The listing builds one solid part. Answer for the finished solid, in the listing's coordinates (mm). A direction names the side the tool comes from. Give positions to 0.01 mm unless a question says otherwise; leave off trailing zeros. Loops run counter-clockwise (first coordinate to the right, second up) from the corner with the lowest first, then second, coordinate; pieces in that order, holes last. Notation, with made-up numbers: (-15.5, -39) -> (43.5, -39) arc R20 cw to (43.5, -23) -> close; hole circle Ø11 at (-30, -15.5). An arc over 180 degrees is marked (long way). One line per question, with ' | ' between items. Start each with the question number.
from build123d import *

# Parameters (mm, degrees)
F1_DEPTH = 10
F2_R     = 10
F3_DEPTH = 10


with BuildPart() as f1:
    # F0 (on Front) → F1 (new body)
    with BuildSketch(Plane.XZ):
        Polygon((0, 10), (0, 0), (60, 0), (60, 10), (26.784621, 10), align=None)
        with BuildLine():
            ThreePointArc((23.443592, 24.368972), (23.75282, 16.867964), (26.784621, 10))
            Line((26.784621, 10), (60, 10))
            ThreePointArc((60, 10), (50.768452, 40.200275), (23.443592, 24.368972))
        make_face()
        with BuildLine():
            Line((0, 30), (0, 10))
            Line((0, 10), (26.784621, 10))
            ThreePointArc((26.784621, 10), (23.75282, 16.867964), (23.443592, 24.368972))
            ThreePointArc((23.443592, 24.368972), (15.503914, 24.276899), (10, 30))
            Line((10, 30), (0, 30))
        make_face()
    extrude(amount=F1_DEPTH)

    # F2 (on face) → F3 (cut)
    with BuildSketch(Plane.XZ.offset(10)):
        with Locations((43.884981, 25.819998)):
            Circle(F2_R)
    extrude(amount=-F3_DEPTH, mode=Mode.SUBTRACT)


solid = f1.part
1. Straight lines are drawn through the part: L1, parallel to X at y = -7.25, z = 27.5; L2, parallel to X at y = -1, z = 21; L3, parallel to X at y = -2.75, z = 31.5. For each, find the intervals that lie inside material, in ascending order.
2. The part is cut by section C-C (z = 6). Write down the section's boundary in (x, y).
3. The part is cut by section B-B (y = -8). Write down the section's boundary in (x, z), plus the area to 3 significant figures.
4. Determine the mould class of faces 1 (the cylindrical face through (15.61, -4.93, 24.233)), 2 (the cylindrical face through (51.24, -4.93, 40.01)), 3 (the flat face through (31, 0, 16)), 4 (the cylindrical face through (48.5, -5.07, 16.95)) for opening direction Z: released by +Z, released by -Z, zero draft, split by the parting line, or undercut.
5. Each of these flat-tipped pins is pushed along its axis until it touches: pin 1 Ø5 at (x, y) = (10, -7) entering from +Z; pin 2 Ø4 at (y, z) = (-7, 30) entering from +X. Where does it stop, or does it pass through?
6. The part is cut by section D-D (x = 4). Write down the section's boundary in (y, z), plus the area to 3 significant figures.
7. The part is cut by section A-A (x = 40). Write down the section's boundary in (y, z).
8. For faces 5 (the flat face through (30, -5, 0)), 6 (the flat face through (5, -5, 30)), 7 (the flat face through (60, -5, 5)), determine the directions among +Z, -Z, +X, -X, +Y, -Y from which every point of the face is accessible in a straight line to the end or side of a thin tool.
Check sheet entries:
1) L1: x = 0 to 11.37, 24.16 to 34.03, 53.74 to 62.62 | L2: x = 0 to 35.12, 52.65 to 63.55 | L3: x = 25.92 to 35.65, 52.12 to 60.86
2) outline: (0, -10) -> (60, -10) -> (60, 0) -> (0, 0) -> close
3) outline: (0, 0) -> (60, 0) -> (60, 10) arc R20.16 ccw (long way) to (23.44, 24.37) arc R10 cw to (10, 30) -> (0, 30) -> close; hole circle Ø20 at (43.88, 25.82) | area: 1,770 mm^2
4) face 1: released by +Z | face 2: split by the parting line | face 3: zero draft | face 4: undercut
5) pin 1: stops at z = 30 | pin 2: stops at x = 62.46
6) outline: (-10, 0) -> (0, 0) -> (0, 30) -> (-10, 30) -> close | area: 300 mm^2
7) outline: (-10, 0) -> (0, 0) -> (0, 16.61) -> (-10, 16.61) -> close; (-10, 35.03) -> (0, 35.03) -> (0, 41.31) -> (-10, 41.31) -> close
8) face 5: -Z, +X, -X, +Y, -Y | face 6: +Z, -X, +Y, -Y | face 7: -Z, +X, +Y, -Y
